Here's the drawing with two shaded views (mm, measured from the low corner). I have some questions. A direction names the side the tool comes from. Round coordinates to 2 decimals unless told otherwise and drop trailing zeros. Loops run counter-clockwise (first coordinate to the right, second up) from the corner with the lowest first, then second, coordinate; pieces in that order, holes last. Notation, with made-up numbers: (2, 17.5) -> (46, 17.5) arc R20 cw to (46, 21.5) -> close; hole circle Ø4 at (-16.5, -26.75). An arc over 180 degrees is marked (long way). Write each question's results on one line, items separated by ' | '. Start each with the question number.
1) For P1, Ø15, axis at x = 79.5, z = 22.5, coming from the +Y side; P2, Ø6, axis at x = 64, y = 14.5, coming from the +Z side; P3, Ø10, axis at x = 67.5, y = 3, coming from the +Z side (1 decimal), each with a flat end and sliding along its axis, tell me the tip position at first contact or that it passes through.
2) Which directions (+Z, -Z, +X, -X, +Y, -Y) give clear straight access to the entire face, cutting with the end or side of a thin tool? Please do the marked faces 4, 5, 6 and 7.
3) Imagine slicing it at B-B, the plane y = 19.4. List the corners of the cut face in (x, z) for me.
4) We'd pull the mould along X, two halves only. Please class the marked faces 1, 2 and 3: pulls with the +X half, pulls with the -X half, needs draft (parallel to the pull), parting line crosses it, or undercut.
5) Imagine slicing it at A-A, the plane y = 6. Give the number of separate pieces and of enclosed holes in the cut face, plus the area to 3 significant figures.
6) Imagine slicing it at D-D, the plane z = 18. List the corners of the cut face in (x, y) for me (1 decimal).
7) If I drill on probe 1 along Y at (x, z) = (89, 6.25); probe 2 along X at (y, z) = (1.75, 17) (1 decimal); probe 3 along Z at (x, y) = (12, 22.5), over which ranges is the centre line in solid material (lowest first)?
8) Imagine slicing it at C-C, the plane x = 15. List the corners of the cut face in (y, z) for me (1 decimal), plus the area to 3 significant figures.
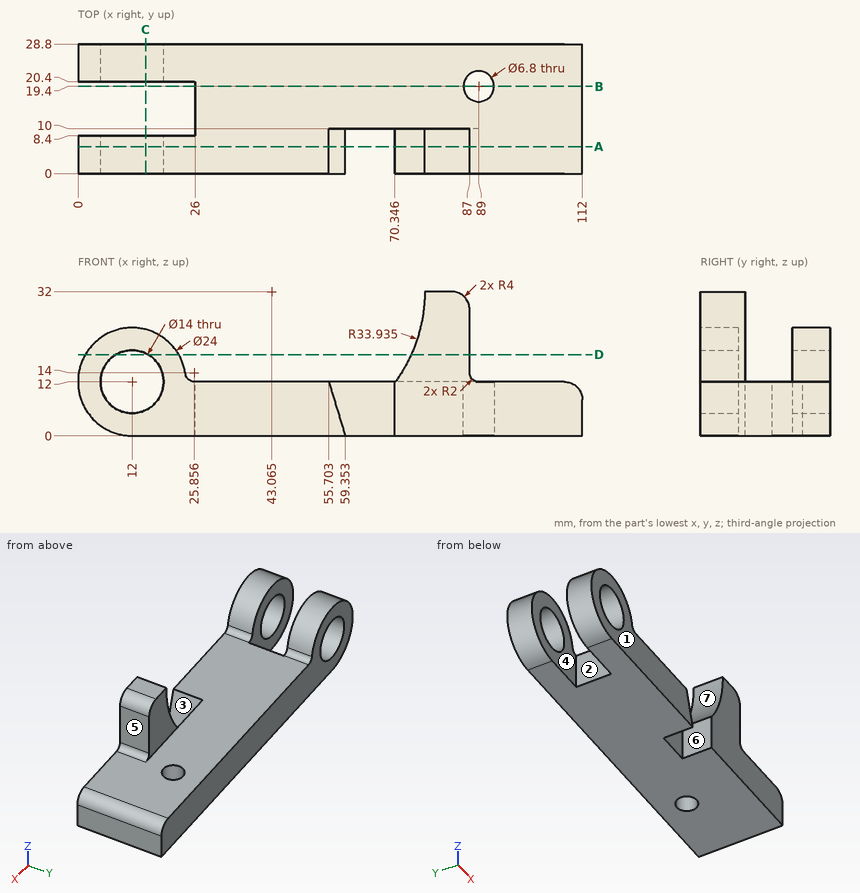
Checked values:
1) P1: y = 10 | P2: z = 12 | P3: z = 15.1
2) face 4: +Z, -Z, -X | face 5: +Z, +X, +Y, -Y | face 6: +Z, -Z, -Y | face 7: +Z, +Y, -Y
3) outline: (26, 0) -> (85.6, 0) -> (85.6, 12) -> (26, 12) -> close; (92.4, 0) -> (112, 0) -> (112, 8) arc R4 ccw to (108, 12) -> (92.4, 12) -> close
4) face 1: needs draft | face 2: pulls with the -X half | face 3: undercut
5) separate pieces: 2 | enclosed holes: 1 | area: 1,470 mm^2
6) outline: (1.6, 0) -> (8.4, 0) -> (8.4, 8.4) -> (1.6, 8.4) -> close; (1.6, 20.4) -> (8.4, 20.4) -> (8.4, 28.8) -> (1.6, 28.8) -> close; (15.6, 0) -> (22.4, 0) -> (22.4, 8.4) -> (15.6, 8.4) -> close; (15.6, 20.4) -> (22.4, 20.4) -> (22.4, 28.8) -> (15.6, 28.8) -> close; (74, 0) -> (87, 0) -> (87, 10) -> (74, 10) -> close
7) probe 1: 0 to 16, 22.8 to 28.8 | probe 2: 1.1 to 7.1, 16.9 to 22.9, 73.5 to 87 | probe 3: 0 to 5, 19 to 24
8) outline: (0, 0) -> (8.4, 0) -> (8.4, 5.7) -> (0, 5.7) -> close; (0, 18.3) -> (8.4, 18.3) -> (8.4, 23.6) -> (0, 23.6) -> close; (20.4, 0) -> (28.8, 0) -> (28.8, 5.7) -> (20.4, 5.7) -> close; (20.4, 18.3) -> (28.8, 18.3) -> (28.8, 23.6) -> (20.4, 23.6) -> close | area: 184 mm^2
